Geometry: final body of the model. Coordinates: model frame, mm. A direction names the side the tool comes from. Give positions to 0.01 mm unless a question says otherwise; leave off trailing zeros. Loops run counter-clockwise (first coordinate to the right, second up) from the corner with the lowest first, then second, coordinate; pieces in that order, holes last.
from build123d import *

# Parameters (mm, degrees)
ESQUISSE1_R                  = 18.9
BOSS_EXTRU_1_DEPTH           = 35.6
BOSS_EXTRU_1_DEPTH_BACK      = 0.1
ESQUISSE3_R                  = 10
BOSS_EXTRU_3_DEPTH           = 4.9
ESQUISSE4_R                  = 3.05
BOSS_EXTRU_4_DEPTH           = 12
ESQUISSE5_R                  = 1.5
ENL_V_MAT_EXTRU_1_DEPTH      = 8
ESQUISSE6_R                  = 7.575
ESQUISSE6_R_2                = 3.05
ENL_V_MAT_EXTRU_3_DEPTH      = 0.65
ENL_V_MAT_EXTRU_4_DEPTH      = 9.6
R_P_TITION_CIRCULAIRE1_COUNT = 3
ESQUISSE8_W                  = 0.25
ESQUISSE8_H                  = 3.196164938


with BuildPart() as part:
    # Esquisse1 → Boss.-Extru.1 (new body, two sides)
    with BuildSketch(Plane.XY) as boss_extru_1_sk:
        Circle(ESQUISSE1_R)
    extrude(amount=BOSS_EXTRU_1_DEPTH)
    extrude(boss_extru_1_sk.sketch, amount=-BOSS_EXTRU_1_DEPTH_BACK)

    # Esquisse3 → Boss.-Extru.3 (add)
    with BuildSketch(Plane.XY.offset(35.6)):
        Circle(ESQUISSE3_R)
    extrude(amount=BOSS_EXTRU_3_DEPTH)

    # Esquisse4 → Boss.-Extru.4 (add)
    with BuildSketch(Plane.XY.offset(40.5)):
        Circle(ESQUISSE4_R)
    extrude(amount=BOSS_EXTRU_4_DEPTH)

    # Esquisse5 → Enlèv. mat.-Extru.1 (cut)
    with BuildSketch(Plane.XY.offset(35.6)):
        with Locations((0, 14.9)):
            Circle(ESQUISSE5_R)
    enl_v_mat_extru_1 = extrude(amount=-ENL_V_MAT_EXTRU_1_DEPTH, mode=Mode.SUBTRACT)

    # Esquisse6 → Enlèv. mat.-Extru.3 (cut)
    with BuildSketch(Plane.XY.offset(40.5)):
        Circle(ESQUISSE6_R)
        Circle(ESQUISSE6_R_2, mode=Mode.SUBTRACT)
    extrude(amount=-ENL_V_MAT_EXTRU_3_DEPTH, mode=Mode.SUBTRACT)

    # Esquisse7 → Enlèv. mat.-Extru.4 (cut)
    with BuildSketch(Plane.XY.offset(52.5)):
        Polygon((-4.317069663, 2.45), (4.517863601, 2.45), (1.480855292, 5.48700831), (-3.363298459, 5.48700831), align=None)
    extrude(amount=-ENL_V_MAT_EXTRU_4_DEPTH, mode=Mode.SUBTRACT)

    # Répétition circulaire1: Enlèv. mat.-Extru.1 ×3 about axis
    r_p_tition_circulaire1_axis = Axis((0, 0, 0), (0, 0, 1))
    for i in range(1, R_P_TITION_CIRCULAIRE1_COUNT):
        add(enl_v_mat_extru_1.rotate(r_p_tition_circulaire1_axis, i * 360 / R_P_TITION_CIRCULAIRE1_COUNT), mode=Mode.SUBTRACT)

    # Esquisse8 → Enlèvement de matière-Révolution1 (revolve, cut)
    with BuildSketch(Plane(origin=(0, 0, 0), x_dir=(0, 0, -1), z_dir=(1, 0, 0))):
        with Locations((-32.675, 20.248082469)):
            Rectangle(ESQUISSE8_W, ESQUISSE8_H)
    revolve(axis=Axis((0, 0, -0.1), (0, 0, 1)), mode=Mode.SUBTRACT)


solid = part.part
Item 1: Section query B-B on x = -13. Return loops of the section in (y, z), plus the area to 3 significant figures.
Values follow:
outline: (-13.72, -0.1) - (13.72, -0.1) - (13.72, 32.55) - (13.37, 32.55) - (13.37, 32.8) - (13.72, 32.8) - (13.72, 35.6) - (-5.95, 35.6) - (-5.95, 27.6) - (-8.95, 27.6) - (-8.95, 35.6) - (-13.72, 35.6) - (-13.72, 32.8) - (-13.37, 32.8) - (-13.37, 32.55) - (-13.72, 32.55) - close
area: 955 mm2
Item 2: Section query A-A on y = 14.9. Return loops of the section in (x, z).
Values follow:
outline: (-11.63, -0.1) - (11.63, -0.1) - (11.63, 32.55) - (11.22, 32.55) - (11.22, 32.8) - (11.63, 32.8) - (11.63, 35.6) - (1.5, 35.6) - (1.5, 27.6) - (-1.5, 27.6) - (-1.5, 35.6) - (-11.63, 35.6) - (-11.63, 32.8) - (-11.22, 32.8) - (-11.22, 32.55) - (-11.63, 32.55) - close
Item 3: Set-up query: faces 1 (the face through (-6.01, -4.61, 40.18)), 2 (the face through (18.027, 5.677, 34.22)). Return all of +Z, -Z, +X, -X, +Y, -Y with unobstructed straight access to the full face (end or side cutting, diameter ignored); none if empty.
Values follow:
face 1: +Z
face 2: +Z, -Z
Item 4: Pin query (flat end, axial travel): pin 1 (10 mm diameter, centred on x = -1, z = 17, fed in from -Y); pin 2 (10 mm diameter, centred on x = -4.5, y = -4, fed in from +Z); pin 3 (1.5 mm diameter, centred on x = 0, y = 15.5, fed in from +Z); pin 4 (3 mm diameter, centred on y = -9, z = 9, fed in from -X). Return the tip coordinate at first contact, or that it passes through.
Values follow:
pin 1: stops at y = -18.9
pin 2: stops at z = 52.5
pin 3: stops at z = 27.6
pin 4: stops at x = -17.35
Item 5: Section query C-C on z = 39. Return loops of the section in (x, y).
Values follow:
outline: circle Ø20 at (0, 0)
Item 6: Draft query along X for faces 3 (the face through (-2.17, -9.76, 38.02)), 4 (the face through (-13, -7, 27.6)), 5 (the face through (0, 2.45, 48)). Return one class per face: +X half, -X half, draft (parallel to the pull), parting line (faces both ways), or undercut.
Values follow:
face 3: parting line
face 4: undercut
face 5: draft
Item 7: Ray query, probe 1 along Y at (x, z) = (0, 40.4) (3 decimals); probe 2 along X at (y, z) = (-7, 29); probe 3 along Y at (x, z) = (0, 30.5). Return the intervals inside material, ascending.
Values follow:
probe 1: y = -10 to -7.575, -3.05 to 3.05, 7.575 to 10
probe 2: x = -17.56 to -14.33, -11.47 to 11.47, 14.33 to 17.56
probe 3: y = -18.9 to 13.4, 16.4 to 18.9
Item 8: Section query D-D on z = 28.5. Return loops of the section in (x, y), plus the area to 3 significant figures.
Values follow:
outline: circle Ø37.8 at (0, 0); hole circle Ø3 at (-12.9, -7.45); hole circle Ø3 at (0, 14.9); hole circle Ø3 at (12.9, -7.45)
area: 1,100 mm2
